from build123d import *

# Parameters (mm, degrees)
SKETCH1_W           = 128.6
SKETCH1_H           = 25
SKETCH1_R           = 1.5
BOSS_EXTRUDE1_DEPTH = 1.6
SKETCH3_W           = 100
SKETCH3_H           = 25
BOSS_EXTRUDE4_DEPTH = 2.54
SKETCH4_W           = 9
SKETCH4_H           = 9
SKETCH4_R           = 1.5
BOSS_EXTRUDE5_DEPTH = 4
FILLET1_R           = 2
SKETCH5_W           = 47.778525573
SKETCH5_H           = 5.095389146
SKETCH5_W_2         = 14.785547181
SKETCH5_H_2         = 6.451421921
CUT_EXTRUDE1_DEPTH  = 67.808679077
FILLET2_R           = 1.5


with BuildPart() as part:
    # Sketch1 → Boss-Extrude1 (new body)
    with BuildSketch(Plane(origin=(0, 0, 0), x_dir=(1, 0, 0), z_dir=(0, 1, 0))):
        Rectangle(SKETCH1_W, SKETCH1_H)
        with Locations(Location((-61.25, -5, 0), (0, 0, 270))):
            Circle(SKETCH1_R, mode=Mode.SUBTRACT)
        with Locations(Location((61.25, -5, 0), (0, 0, 270))):
            Circle(SKETCH1_R, mode=Mode.SUBTRACT)
    extrude(amount=BOSS_EXTRUDE1_DEPTH)

    # Sketch3 → Boss-Extrude4 (add)
    with BuildSketch(Plane(origin=(0, 0, 0), x_dir=(1, 0, 0), z_dir=(0, 1, 0))):
        Rectangle(SKETCH3_W, SKETCH3_H)
    extrude(amount=-BOSS_EXTRUDE4_DEPTH)

    # Sketch4 → Boss-Extrude5 (add)
    # profile 1 of 2: a face of its own
    with BuildSketch(Plane.XY.offset(8.5)):
        with Locations((-45.5, -7.04)):
            Rectangle(SKETCH4_W, SKETCH4_H)
        with Locations((-44.5, -6.08)):
            Circle(SKETCH4_R, mode=Mode.SUBTRACT)
    # profile 2 of 2: a face of its own
    with BuildSketch(Plane.XY.offset(8.5)):
        with Locations((45.5, -7.04)):
            Rectangle(SKETCH4_W, SKETCH4_H)
        with Locations((44.5, -6.08)):
            Circle(SKETCH4_R, mode=Mode.SUBTRACT)
    extrude(amount=-BOSS_EXTRUDE5_DEPTH)

    # Fillet1
    fillet1_edges = [part.edges().sort_by_distance(p)[0] for p in [
        (-45.5, -2.54, 4.5),
        (45.5, -2.54, 4.5),
    ]]
    fillet(fillet1_edges, radius=FILLET1_R)

    # Sketch5 → Cut-Extrude1 (cut, through all)
    with BuildSketch(Plane(origin=(0, 1.6, 0), x_dir=(1, 0, 0), z_dir=(0, 1, 0))):
        with Locations((15.567152962, -5.952305427)):
            Rectangle(SKETCH5_W, SKETCH5_H)
        with Locations((-24.988389969, -1.104696386)):
            Rectangle(SKETCH5_W_2, SKETCH5_H_2)
    extrude(amount=-CUT_EXTRUDE1_DEPTH, mode=Mode.SUBTRACT)

    # Fillet2
    fillet2_edges = [part.edges().sort_by_distance(p)[0] for p in [
        (-24.988389969, 1.6, 4.330407346),
        (-17.595616378, 1.6, 1.104696385),
        (-24.988389969, 1.6, -2.121014575),
        (-8.322109824, 1.6, 5.952305427),
        (15.567152962, 1.6, 8.5),
        (39.456415749, 1.6, 5.952305427),
        (15.567152962, 1.6, 3.404610854),
        (-32.381163559, 1.6, 1.104696385),
    ]]
    fillet(fillet2_edges, radius=FILLET2_R)


solid = part.part
Check sheet for the modelled part. Datum: model origin and axes. Units: mm. A direction names the side the tool comes from. Give positions to 0.01 mm unless a question says otherwise; leave off trailing zeros. Write each loop counter-clockwise with the first axis right and the second up, starting at its lowest first coordinate (ties: lowest second). Pieces come first, ordered by that corner, then holes. Notation, with made-up numbers: (12, -5) -> (34, -5) arc R32 ccw to (34, 28) -> close; hole circle Ø10 at (47.25, -1). An arc over 180 degrees is marked (long way). One line per item, written item: value. Start each with the question number.
Item 1: Gauge pin test, flat ends, axial feed: pin 1 (11.5 mm diameter, centred on x = 57, z = -4.5, fed in from -Y); pin 2 (2.5 mm diameter, centred on x = 46.5, y = -8, fed in from +Z); pin 3 (1.3 mm diameter, centred on y = -1.5, z = 1, fed in from -X). Record the tip position at first contact, or that the pin passes through.
Item 2: Section check B-B on x = -44.5. Record the cut outline in (y, z).
Item 3: Section check A-A on y = -6.08. Record the cut outline in (x, z), then the cut area to 3 significant figures.
Item 4: Material ranges on probe 1 along X at (y, z) = (-1.75, 3.5); probe 2 along Z at (x, y) = (29, 0); probe 3 along X at (y, z) = (-0.75, 0.25), recorded low to high. Write a range as from..to.
Item 5: Section check D-D on y = -1.25. Record the cut outline in (x, z).
Item 6: Tool access check on faces 5 (the flat face through (-17.596, -1, 1)), 6 (the flat face through (50, -2.8, 3.8)), 7 (the flat face through (-46, -8, 4.5)), 8 (the flat face through (-41, -7, 6)), 9 (the flat face through (45, -8, 8.5)). Record the directions out of +Z, -Z, +X, -X, +Y, -Y that give a thin tool (end or side, any length) a straight path to the whole face; none if there is none.
Item 7: Section check C-C on z = 0.75. Record the cut outline in (x, y).
Item 8: Draft check along Y on faces 1 (the flat face through (-46, -11.54, 7)), 2 (the cylindrical face through (43, -6.01, 6.53)), 3 (the cylindrical face through (-46, -6.01, 6.53)), 4 (the flat face through (-47, -7, 8.5)). Enter one of: +Y half, -Y half, draft (parallel to the pull), parting line (faces both ways), or undercut.
Results list:
1. pin 1: y = 0
1. pin 2: z = 8.5
1. pin 3: x = -50
2. outline: (-11.54, 4.5) -> (-7.58, 4.5) -> (-7.58, 8.5) -> (-11.54, 8.5) -> close; (-4.58, 4.5) -> (-4.54, 4.5) arc R2 cw to (-2.54, 2.5) -> (-2.54, -12.5) -> (1.6, -12.5) -> (1.6, 12.5) -> (-2.54, 12.5) -> (-2.54, 8.5) -> (-4.58, 8.5) -> close
3. outline: (-50, 4.5) -> (-46, 4.5) -> (-46, 8.5) -> (-50, 8.5) -> close; (-43, 4.5) -> (-41, 4.5) -> (-41, 8.5) -> (-43, 8.5) -> close; (41, 4.5) -> (43, 4.5) -> (43, 8.5) -> (41, 8.5) -> close; (46, 4.5) -> (50, 4.5) -> (50, 8.5) -> (46, 8.5) -> close
3. area: 48.0 mm²
4. probe 1: -50..-32.38, -17.6..-8.32, 39.46..50
4. probe 2: -12.5..3.4, 8.5..12.5
4. probe 3: -50..-32.38, -17.6..50
5. outline: (-50, -12.5) -> (50, -12.5) -> (50, 12.5) -> (-50, 12.5) -> close; hole (-32.38, -2.12) -> (-17.6, -2.12) -> (-17.6, 4.33) -> (-32.38, 4.33) -> close; hole (-8.32, 3.4) -> (39.46, 3.4) -> (39.46, 8.5) -> (-8.32, 8.5) -> close
6. face 5: +Y, -Y
6. face 6: +Z, -Z, +X, -Y
6. face 7: -Z, +X, -X, -Y
6. face 8: +Z, -Z, -Y
6. face 9: +Z, +X, -X, -Y
7. outline: (-64.3, 0) -> (-50, 0) -> (-50, -2.54) -> (-32.38, -2.54) -> (-32.38, 0.1) arc R1.5 ccw to (-33.88, 1.6) -> (-64.3, 1.6) -> close; (-17.6, -2.54) -> (50, -2.54) -> (50, 0) -> (64.3, 0) -> (64.3, 1.6) -> (-16.1, 1.6) arc R1.5 ccw to (-17.6, 0.1) -> close
8. face 1: -Y half
8. face 2: undercut
8. face 3: undercut
8. face 4: draft
